from build123d import *

# Parameters (mm, degrees)
F1_DEPTH = 10.16


with BuildPart() as f1:
    # F0 (on Top) → F1 (new body, symmetric)
    with BuildSketch(Plane.XY):
        Polygon((18.139582, 56.243164), (-26.708071, 76.492655), (-37.614409, 69.445336), (-37.614409, -57.554664), (-29.616961, -65.016977), (19.900086, -42.659173), (23.599582, -36.426205), (23.599582, 48.777979), align=None)
        Polygon((-29.616961, -57.554664), (-29.616961, 69.445336), (16.682325, 48.540407), (16.682325, -36.649735), align=None, mode=Mode.SUBTRACT)
    extrude(amount=F1_DEPTH, both=True)


solid = f1.part
The listing builds one solid part. Answer for the finished solid, in the listing's coordinates (mm). A direction names the side the tool comes from. Give positions to 0.01 mm unless a question says otherwise; leave off trailing zeros. Order: outer loops, then holes, each group sorted by start corner. A loop starts at its lowest first (then second) coordinate and runs counter-clockwise, first axis right, second up. Notation, with made-up numbers: (37.5, -5) - (72.5, -5) arc R21 cw to (72.5, 1) - close; hole circle Ø9 at (-24, -28). An arc over 180 degrees is marked (long way). One line per item, written item: value. Start each with the question number.
1) A cutting plane is placed at A-A on z = -2.5. Give the vertices of the cut face in (x, y), then the cut area to 3 significant figures.
2) A tool of negligible diameter and unlimited length cuts with its end or side. For faces 1 (the face through (-6.143, -46.956, 0.142)), 2 (the face through (-33.672, -61.234, 0.142)), from which of +Z, -Z, +X, -X, +Y, -Y can it reach the whole face along a straight path? Write none if from no direction.
3) A cutting plane is placed at C-C on x = -28. Give the vertices of the cut face in (y, z).
4) The mould has two halves that part along X. Classify faces 3 (the face through (21.72, -39.59, 0.14)), 4 (the face through (-6.79, 59.14, 0.14)), 5 (the face through (-30, 11, -10.16)), 6 (the face through (-29.617, 5, 0)): released by +X, released by -X, zero draft, split by the parting line, or undercut.
5) A cutting plane is placed at B-B on y = 15. Give the vertices of the cut face in (x, z), then the cut area to 3 significant figures.
6) Find the intervals of material crossed by L1, parallel to X at y = 39.5, z = -4.75; L2, parallel to Y at x = -9, z = -3; L3, parallel to X at y = 64.5, z = -7.5, in increasing order.
7) Given pin 1 Ø1.5 at (x, z) = (-2.5, 4) entering from +Y; pin 2 Ø3 at (x, z) = (16.5, 3.5) entering from +Y, each flat-ended and moving along its own axis, determine where each tip first touches the part or whether it passes through.
Answer sheet:
1. outline: (-37.61, -57.55) - (-29.62, -65.02) - (19.9, -42.66) - (23.6, -36.43) - (23.6, 48.78) - (18.14, 56.24) - (-26.71, 76.49) - (-37.61, 69.45) - close; hole (-29.62, -57.55) - (16.68, -36.65) - (16.68, 48.54) - (-29.62, 69.45) - close
1. area: 2,450 mm2
2. face 1: +Z, -Z
2. face 2: +Z, -Z, -X, -Y
3. outline: (-64.29, -10.16) - (-56.82, -10.16) - (-56.82, 10.16) - (-64.29, 10.16) - close; (68.72, -10.16) - (75.66, -10.16) - (75.66, 10.16) - (68.72, 10.16) - close
4. face 3: released by +X
4. face 4: undercut
4. face 5: zero draft
4. face 6: undercut
5. outline: (-37.61, -10.16) - (-29.62, -10.16) - (-29.62, 10.16) - (-37.61, 10.16) - close; (16.68, -10.16) - (23.6, -10.16) - (23.6, 10.16) - (16.68, 10.16) - close
5. area: 303 mm2
6. L1: x = -37.61 to -29.62, 16.68 to 23.6
6. L2: y = -55.71 to -48.25, 60.14 to 68.5
6. L3: x = -37.61 to -29.62, -18.66 to -0.15
7. pin 1: stops at y = 65.9
7. pin 2: stops at y = 57.66
